The listing builds one solid part. Answer for the finished solid, in the listing's coordinates (mm). Give positions to 0.01 mm unless a question says otherwise; leave off trailing zeros. Order: outer loops, then holes, each group sorted by start corner. A loop starts at its lowest first (then second) coordinate and runs counter-clockwise, first axis right, second up. Notation, with made-up numbers: (8.5, 54) - (49.5, 54) arc R14 ccw to (49.5, 58) - close; hole circle Ø8 at (86.25, 6). An arc over 180 degrees is marked (long way). Use a Markdown table: item, result. Add a question column.
1) Straight lines are drawn through the part: line 1 (Z direction, x = 3.25, y = 80); line 2 (Y direction, x = 1.2, z = -311); line 3 (Z direction, x = 1.5, y = 8.5). For each, find the intervals that lie inside material, in ascending order.
2) Find section B-B, the plane z = -10. Determine the outline of the cut face in (x, y).
3) Find section A-A, the plane y = 30. Determine the outline of the cut face in (x, z).
from build123d import *

# Parameters (mm, degrees)
SKETCH_1_W      = 350
SKETCH_1_H      = 85
SKETCH_1_R      = 2.95
SKETCH_1_R_2    = 1.45
EXTRUDE_1_DEPTH = 4
FILLET_1_R      = 1


with BuildPart() as part:
    # 草图1 → 凸台-拉伸1 (new body)
    with BuildSketch(Plane(origin=(0, 0, 0), x_dir=(0, 0, -1), z_dir=(1, 0, 0))):
        with Locations((175, 42.5)):
            Rectangle(SKETCH_1_W, SKETCH_1_H)
        with Locations((10, 30)):
            Circle(SKETCH_1_R, mode=Mode.SUBTRACT)
        with Locations((10, 10)):
            Circle(SKETCH_1_R, mode=Mode.SUBTRACT)
        with Locations((15, 80)):
            Circle(SKETCH_1_R_2, mode=Mode.SUBTRACT)
        with Locations((39, 80)):
            Circle(SKETCH_1_R_2, mode=Mode.SUBTRACT)
        with Locations((15, 50)):
            Circle(SKETCH_1_R_2, mode=Mode.SUBTRACT)
        with Locations((39, 50)):
            Circle(SKETCH_1_R_2, mode=Mode.SUBTRACT)
        with Locations(Location((311, 50, 0), (0, 0, 180))):
            Circle(SKETCH_1_R_2, mode=Mode.SUBTRACT)
        with Locations(Location((335, 50, 0), (0, 0, 180))):
            Circle(SKETCH_1_R_2, mode=Mode.SUBTRACT)
        with Locations(Location((311, 80, 0), (0, 0, 180))):
            Circle(SKETCH_1_R_2, mode=Mode.SUBTRACT)
        with Locations(Location((335, 80, 0), (0, 0, 180))):
            Circle(SKETCH_1_R_2, mode=Mode.SUBTRACT)
        with Locations(Location((340, 10, 0), (0, 0, 180))):
            Circle(SKETCH_1_R, mode=Mode.SUBTRACT)
        with Locations(Location((340, 30, 0), (0, 0, 180))):
            Circle(SKETCH_1_R, mode=Mode.SUBTRACT)
    extrude(amount=EXTRUDE_1_DEPTH)

    # 圆角1
    fillet_1_edges = [part.edges().sort_by_distance(p)[0] for p in [
        (2, 85, 0),
        (2, 85, -350),
        (2, 0, -350),
        (2, 0, 0),
    ]]
    fillet(fillet_1_edges, radius=FILLET_1_R)


solid = part.part
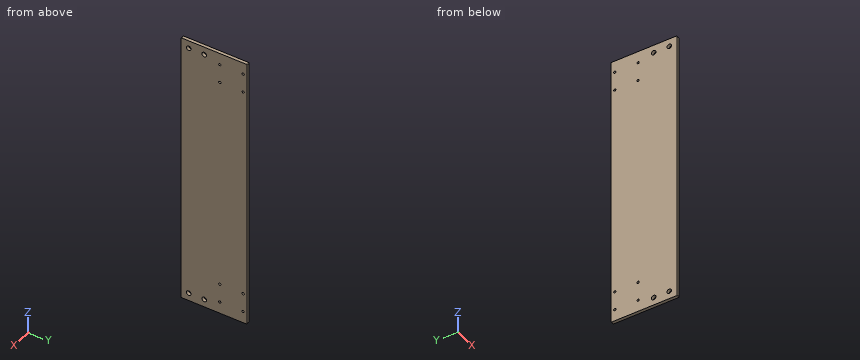
The answers:
| question | item | result |
|---|---|---|
| 1 | line 1 | -350 to -336.45, -333.55 to -312.45, -309.55 to -40.45, -37.55 to -16.45, -13.55 to 0 |
| 1 | line 2 | 0 to 48.55, 51.45 to 78.55, 81.45 to 85 |
| 1 | line 3 | -350 to -342.54, -337.46 to -12.54, -7.46 to 0 |
| 2 | outline | (0, 0) - (4, 0) - (4, 7.05) - (0, 7.05) - close; (0, 12.95) - (4, 12.95) - (4, 27.05) - (0, 27.05) - close; (0, 32.95) - (4, 32.95) - (4, 85) - (0, 85) - close |
| 3 | outline | (0, -350) - (4, -350) - (4, -342.95) - (0, -342.95) - close; (0, -337.05) - (4, -337.05) - (4, -12.95) - (0, -12.95) - close; (0, -7.05) - (4, -7.05) - (4, 0) - (0, 0) - close |
